Can you work these out from the model? Positions are in its coordinate system, mm. Coordinates: 2 decimals unless noted, no trailing zeros. Order: outer loops, then holes, each group sorted by start corner. A loop starts at its lowest first (then second) coordinate and runs counter-clockwise, first axis right, second up. Notation, with made-up numbers: M -16.5,82 L -2.5,82 A26 ccw -2.5,116 Z; hole C -19.75,-40 d7. An arc over 180 degrees is marked long. Answer as a JSON object with one key per item and string values.
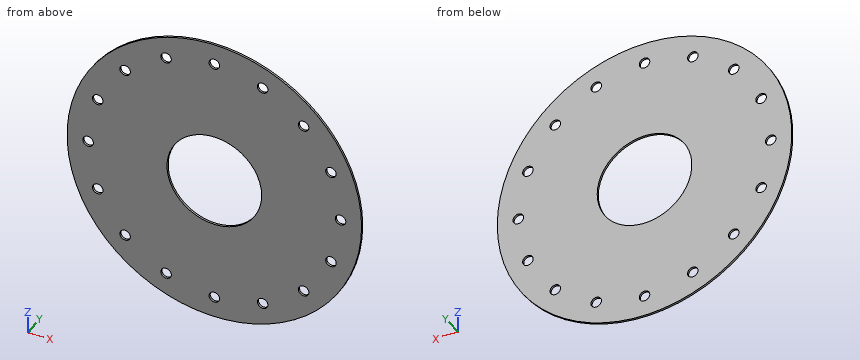
Autodesk Fusion 360 part; units mm, degrees
sketch "Sketch1" plane through (0, 0, 0) normal (0, 1, 0) x (1, 0, 0)
  circle A0 centre (0, 0) radius 60 construction
  circle A1 centre (0, 0) radius 22.5
  circle A2 centre (0, 0) radius 70
  point P0 (-60, 0)
  dimension "d1" = 120
  dimension "d2" = 45
  dimension "d3" = 140
extrude "Extrude1" add sketch "Sketch1" along normal blind 1
hole "Hole1" at (-60, 0, 0) direction (0, 1, 0) diameter 5 depth 30 tip angle 118
pattern_circular "C-Pattern1" count 16 over 360 about axis through (0, 1.75, 0) along (0, 1, 0) of "Hole1"
sketch "cutting pattern" plane through (0, 1, 0) normal (0, 1, 0) x (-1, 0, 0)
  circle A0 centre (55.4328, -22.961) radius 2.5
  circle A1 centre (42.4264, -42.4264) radius 2.5
  circle A2 centre (22.961, -55.4328) radius 2.5
  circle A3 centre (0, -60) radius 2.5
  circle A4 centre (-22.961, -55.4328) radius 2.5
  circle A5 centre (-42.4264, -42.4264) radius 2.5
  circle A6 centre (-55.4328, -22.961) radius 2.5
  circle A7 centre (-60, 0) radius 2.5
  circle A8 centre (-55.4328, 22.961) radius 2.5
  circle A9 centre (-42.4264, 42.4264) radius 2.5
  circle A10 centre (-22.961, 55.4328) radius 2.5
  circle A11 centre (0, 60) radius 2.5
  circle A12 centre (22.961, 55.4328) radius 2.5
  circle A13 centre (42.4264, 42.4264) radius 2.5
  circle A14 centre (55.4328, 22.961) radius 2.5
  circle A15 centre (60, 0) radius 2.5
  circle A16 centre (0, 0) radius 22.5
  circle A17 centre (0, 0) radius 70
Item 1: I want a section at A-A, the plane z = 0. Write out the boundary of the cut face in (x, y), plus the area to 3 significant figures.
Answers follow:
{"outline": "M -70,0 L -62.5,0 L -62.5,1 L -70,1 Z; M -57.5,0 L -22.5,0 L -22.5,1 L -57.5,1 Z; M 22.5,0 L 57.5,0 L 57.5,1 L 22.5,1 Z; M 62.5,0 L 70,0 L 70,1 L 62.5,1 Z", "area": "85.0 mm^2"}
Item 2: I want a section at D-D, the plane z = -60. Write out the boundary of the cut face in (x, y).
Answers follow:
{"outline": "M -36.06,0 L -2.5,0 L -2.5,1 L -36.06,1 Z; M 2.5,0 L 36.06,0 L 36.06,1 L 2.5,1 Z"}
Item 3: I'm going to push a flat-ended pin straight in: pin 1 (8 mm diameter, centred on x = -22.96, z = -55.43, fed in from +Y). Where does the tip first touch, or does it pass through?
Answers follow:
{"pin 1": "stops at y = 1"}
Item 4: I want a section at B-B, the plane x = 15.5. Write out the boundary of the cut face in (y, z).
Answers follow:
{"outline": "M 0,-68.26 L 1,-68.26 L 1,-16.31 L 0,-16.31 Z; M 0,16.31 L 1,16.31 L 1,68.26 L 0,68.26 Z"}
Item 5: Please list where these lines run through material, in increasing order: line 1 (X direction, y = 0.75, z = 42.5); line 2 (X direction, y = 0.3, z = 0); line 3 (Z direction, x = 56, y = 0.5).
Answers follow:
{"line 1": "x = -55.62 to -44.93, -39.93 to 39.93, 44.93 to 55.62", "line 2": "x = -70 to -62.5, -57.5 to -22.5, 22.5 to 57.5, 62.5 to 70", "line 3": "z = -42 to -25.4, -20.53 to 20.53, 25.4 to 42"}
